```python
from build123d import *

# Parameters (mm, degrees)
CROQUIS1_W              = 20.2
CROQUIS1_H              = 48
SALIENTE_EXTRUIR1_DEPTH = 7
CROQUIS2_W              = 7
CROQUIS2_H              = 20.2
CORTAR_EXTRUIR1_DEPTH   = 2.2
CROQUIS3_R              = 1.62
CROQUIS3_R_2            = 1.65
CORTAR_EXTRUIR2_DEPTH   = 15
CROQUIS4_R              = 1.65
CORTAR_EXTRUIR3_DEPTH   = 15
CHAFL_N1_SIZE           = 0.5
REDONDEO1_R             = 5
CROQUIS5_W              = 5
CROQUIS5_H              = 3
CORTAR_EXTRUIR4_DEPTH   = 7
CROQUIS6_W              = 3
CROQUIS6_H              = 2.5
CORTAR_EXTRUIR5_DEPTH   = 7
REDONDEO2_R             = 0.5


with BuildPart() as part:
    # Croquis1 → Saliente-Extruir1 (new body)
    with BuildSketch(Plane(origin=(0, 0, 0), x_dir=(0, 0, -1), z_dir=(1, 0, 0))):
        with Locations((10.1, 24)):
            Rectangle(CROQUIS1_W, CROQUIS1_H)
    extrude(amount=SALIENTE_EXTRUIR1_DEPTH)

    # Croquis2 → Cortar-Extruir1 (cut)
    with BuildSketch(Plane.XY):
        with Locations((3.5, 37.9)):
            Rectangle(CROQUIS2_W, CROQUIS2_H)
    extrude(amount=-CORTAR_EXTRUIR1_DEPTH, mode=Mode.SUBTRACT)

    # Croquis3 → Cortar-Extruir2 (cut)
    with BuildSketch(Plane.XZ):
        with Locations(Location((4.15, -5.1, 0), (0, 0, 270))):
            Circle(CROQUIS3_R)
        with Locations(Location((4.15, -15.1, 0), (0, 0, 270))):
            Circle(CROQUIS3_R_2)
    extrude(amount=-CORTAR_EXTRUIR2_DEPTH, mode=Mode.SUBTRACT)

    # Croquis4 → Cortar-Extruir3 (cut)
    with BuildSketch(Plane.XY.offset(-2.2)):
        with Locations((4.15, 32.9)):
            Circle(CROQUIS4_R)
        with Locations((4.15, 42.9)):
            Circle(CROQUIS4_R)
    extrude(amount=-CORTAR_EXTRUIR3_DEPTH, mode=Mode.SUBTRACT)

    # Chaflán1
    chafl_n1_edges = [part.edges().sort_by_distance(p)[0] for p in [
        (4.15, 0, -3.48),
        (4.15, 0, -13.45),
        (2.5, 42.9, -2.2),
        (2.5, 32.9, -2.2),
    ]]
    chamfer(chafl_n1_edges, length=CHAFL_N1_SIZE)

    # Redondeo1
    redondeo1_edges = [part.edges().sort_by_distance(p)[0] for p in [
        (3.5, 48, -20.2),
    ]]
    fillet(redondeo1_edges, radius=REDONDEO1_R)

    # Croquis5 → Cortar-Extruir4 (cut)
    with BuildSketch(Plane(origin=(7, 0, 0), x_dir=(0, 0, -1), z_dir=(1, 0, 0))):
        with Locations((10.1, 18.5)):
            Rectangle(CROQUIS5_W, CROQUIS5_H)
    extrude(amount=-CORTAR_EXTRUIR4_DEPTH, mode=Mode.SUBTRACT)

    # Croquis6 → Cortar-Extruir5 (cut)
    with BuildSketch(Plane(origin=(7, 0, 0), x_dir=(0, 0, -1), z_dir=(1, 0, 0))):
        with Locations((10.1, 21.25)):
            Rectangle(CROQUIS6_W, CROQUIS6_H)
        with Locations((10.1, 15.75)):
            Rectangle(CROQUIS6_W, CROQUIS6_H)
    extrude(amount=-CORTAR_EXTRUIR5_DEPTH, mode=Mode.SUBTRACT)

    # Redondeo2
    redondeo2_edges = [part.edges().sort_by_distance(p)[0] for p in [
        (3.5, 17, -8.6),
        (3.5, 20, -8.6),
        (3.5, 20, -11.6),
        (3.5, 17, -11.6),
    ]]
    fillet(redondeo2_edges, radius=REDONDEO2_R)


solid = part.part
```
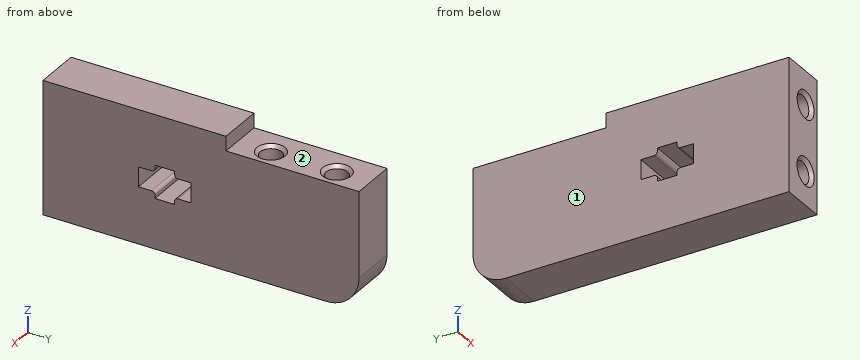
The listing builds one solid part. Answer for the finished solid, in the listing's coordinates (mm). Face numbers are marked on the shaded views. A direction names the side the tool comes from. Round coordinates to 2 decimals unless told otherwise and drop trailing zeros. Order: outer loops, then holes, each group sorted by start corner. A loop starts at its lowest first (then second) coordinate and runs counter-clockwise, first axis right, second up. Notation, with made-up numbers: (-18.5, 62) -> (-9.5, 62) arc R14 cw to (-9.5, 75) -> close; hole circle Ø1 at (-19, 42.5). An arc over 180 degrees is marked (long way). Answer as CSV lines item,"result".
Q1. A cutting plane is placed at C-C on y = 8. Determine the outline of the cut face in (x, z).
Computed values:
outline,"(0, -20.2) -> (7, -20.2) -> (7, 0) -> (0, 0) -> close; hole circle Ø3.3 at (4.15, -15.1); hole circle Ø3.24 at (4.15, -5.1)"
Q2. Consider line 1 (Z direction, x = 4, y = 9.5); line 2 (Y direction, x = 4.15, z = -6.5); line 3 (Y direction, x = 0.75, z = -9.5). Determine where each line is inside the solid, lowest interval first. Write a range as from..to.
Computed values:
line 1,"z = -20.2..-16.74, -13.46..-6.71, -3.49..0"
line 2,"y = 15..31.25, 34.55..41.25, 44.55..48"
line 3,"y = 0..14.5, 22.5..48"
Q3. A cutting plane is placed at D-D on z = -14. Give the number of separate pieces and of enclosed holes in the cut face, plus the area to 3 significant figures.
Computed values:
separate pieces,"1"
enclosed holes,"2"
area,"282 mm^2"
Q4. A cutting plane is placed at B-B on y = 32.9. Determine the outline of the cut face in (x, z).
Computed values:
outline,"(0, -20.2) -> (7, -20.2) -> (7, -2.2) -> (6.3, -2.2) -> (5.8, -2.7) -> (5.8, -17.2) -> (2.5, -17.2) -> (2.5, -2.7) -> (2, -2.2) -> (0, -2.2) -> close"
Q5. A cutting plane is placed at A-A on z = -5.1. Determine the outline of the cut face in (x, y).
Computed values:
outline,"(0, 0) -> (2.03, 0) -> (2.53, 0.5) -> (2.53, 15) -> (5.77, 15) -> (5.77, 0.5) -> (6.27, 0) -> (7, 0) -> (7, 48) -> (0, 48) -> close; hole circle Ø3.3 at (4.15, 32.9); hole circle Ø3.3 at (4.15, 42.9)"
Q6. Which of the six approach directions +Z, -Z, +X, -X, +Y, -Y give full straight-line access (tool end or side, diameter ignored) to the marked faces 1 and 2?
Computed values:
face 1,"+Z, -Z, -X, +Y, -Y"
face 2,"+Z, +X, -X, +Y"
Q7. Given pin 1 (1 mm diameter, centred on x = 3.5, z = -15, fed in from -Y); pin 2 (1.8 mm diameter, centred on x = 5, z = -1, fed in from +Y); pin 3 (1 mm diameter, centred on x = 5, y = 33, fed in from +Z), each flat-ended and moving along its own axis, determine where each tip first touches the part or whether it passes through.
Computed values:
pin 1,"stops at y = 15"
pin 2,"stops at y = 27.8"
pin 3,"stops at z = -17.2"
